The model under review builds one solid part; all positions refer to its coordinate system, in mm. Give positions to 0.01 mm unless a question says otherwise; leave off trailing zeros. Loops run counter-clockwise (first coordinate to the right, second up) from the corner with the lowest first, then second, coordinate; pieces in that order, holes last. Notation, with made-up numbers: M 59.5,47.5 L 71.5,47.5 A7 ccw 71.5,55.5 Z; hole C -28.5,-6.5 d6. An arc over 180 degrees is marked long. Put each result on its own line as item: value. Start each with the question number.
from build123d import *

# Parameters (mm, degrees)
SKETCH1_R           = 2.4892
BOSS_EXTRUDE1_DEPTH = 3.175


with BuildPart() as part:
    # Sketch1 → Boss-Extrude1 (new body)
    with BuildSketch(Plane(origin=(0, 0, 0), x_dir=(1, 0, 0), z_dir=(0, 1, 0))):
        with BuildLine():
            ThreePointArc((-30.1625, 0), (15.08125, -26.121491242), (15.08125, 26.121491242))
            ThreePointArc((15.08125, 26.121491242), (8.575554014, 24.378295256), (10.31875, 17.872599271))
            ThreePointArc((10.31875, 17.872599271), (10.31875, -17.872599271), (-20.6375, 0))
            ThreePointArc((-20.6375, 0), (-25.4, 4.7625), (-30.1625, 0))
        make_face()
        with Locations(Location((25.4, 0, 0), (0, 0, 270))):
            Circle(SKETCH1_R, mode=Mode.SUBTRACT)
        with Locations(Location((21.997045256, -12.7, 0), (0, 0, 270))):
            Circle(SKETCH1_R, mode=Mode.SUBTRACT)
        with Locations(Location((12.7, -21.997045256, 0), (0, 0, 270))):
            Circle(SKETCH1_R, mode=Mode.SUBTRACT)
        with Locations(Location((0, -25.4, 0), (0, 0, 270))):
            Circle(SKETCH1_R, mode=Mode.SUBTRACT)
        with Locations(Location((-12.7, -21.997045256, 0), (0, 0, 270))):
            Circle(SKETCH1_R, mode=Mode.SUBTRACT)
        with Locations(Location((-21.997045256, -12.7, 0), (0, 0, 270))):
            Circle(SKETCH1_R, mode=Mode.SUBTRACT)
        with Locations(Location((-25.4, 0, 0), (0, 0, 270))):
            Circle(SKETCH1_R, mode=Mode.SUBTRACT)
        with Locations(Location((12.7, 21.997045256, 0), (0, 0, 270))):
            Circle(SKETCH1_R, mode=Mode.SUBTRACT)
        with Locations(Location((21.997045256, 12.7, 0), (0, 0, 270))):
            Circle(SKETCH1_R, mode=Mode.SUBTRACT)
    extrude(amount=BOSS_EXTRUDE1_DEPTH)


solid = part.part
(1) We need section D-D, the plane x = 12.7. Write out the cut boundary in (y, z) (3 decimals), plus the area to 3 significant figures.
(2) We need section B-B, the plane z = 18. Write out the cut boundary in (x, y) (3 decimals), plus the area to 3 significant figures.
(3) We need section C-C, the plane y = 0.55. State how many separate pieces and enclosed holes the cut face has, plus the area to 3 significant figures.
(4) We need section A-A, the plane x = -25.4. Write out the cut boundary in (y, z) (1 decimal).
(5) To check wall thickness, follow L1, parallel to Z at x = 14, y = 2; L2, parallel to X at y = 2.4, z = 0.5; L3, parallel to X at y = 2.7, z = 11.5. State the ranges of each line that lie inside material, in increasing order. Write a range as [from, to].
(6) Insertion check: pin 1 (1 mm diameter, centred on x = 10.5, y = 2, fed in from +Z); pin 2 (1.5 mm diameter, centred on y = 1.5, z = -20, fed in from +X). Each pin has a flat end and moves straight along its axis. Give the tip position at first contact, or say it passes through.
(7) Draft analysis for pull direction X (two halves, no side actions). For faces 1 (the cylindrical face through (24.465, 1.565, 12.376)), 2 (the cylindrical face through (13.448, 1.565, -19.623)), 3 (the cylindrical face through (14.31, 1.57, 26.55)), 4 (the flat face through (4, 0, 21)), state which applies: +X half, -X half, draft (parallel to the pull), parting line (faces both ways), or undercut.
Check sheet entries:
1. outline: M 0,-26.76 L 3.175,-26.76 L 3.175,-24.486 L 0,-24.486 Z; M 0,-19.508 L 3.175,-19.508 L 3.175,-16.267 L 0,-16.267 Z; M 0,16.267 L 3.175,16.267 L 3.175,19.508 L 0,19.508 Z; M 0,24.486 L 3.175,24.486 L 3.175,27.358 L 0,27.358 Z
1. area: 36.9 mm²
2. outline: M -24.203,0 L -10.095,0 L -10.095,3.175 L -24.203,3.175 Z; M 10.095,0 L 24.203,0 L 24.203,3.175 L 10.095,3.175 Z
2. area: 89.6 mm²
3. separate pieces: 1
3. enclosed holes: 9
3. area: 909 mm²
4. outline: M 0,-4.8 L 3.2,-4.8 L 3.2,-2.5 L 0,-2.5 Z; M 0,2.5 L 3.2,2.5 L 3.2,16.3 L 0,16.3 Z
5. L1: z = [-26.58, -24.12], [-19.87, -15.16], [15.16, 19.87], [24.12, 26.72]
5. L2: x = [-30.16, -27.84], [-22.96, -20.63], [20.63, 22.96], [27.84, 30.16]
5. L3: x = [-27.88, -24.18], [-19.82, -17.14], [17.14, 19.82], [24.18, 27.88]
6. pin 1: stops at z = 28.46
6. pin 2: stops at x = 23.22
7. face 1: undercut
7. face 2: undercut
7. face 3: parting line
7. face 4: draft
